Autodesk Inventor part; units mm, degrees
ref_plane "YZ Plane" through (0, 0, 0) normal (1, 0, 0) x (0, 1, 0)
ref_plane "XZ Plane" through (0, 0, 0) normal (0, 1, 0) x (-1, 0, 0)
ref_plane "XY Plane" through (0, 0, 0) normal (0, 0, 1) x (1, 0, 0)
sketch "Sketch1" plane through (0, 0, 0) normal (0, 0, 1) x (1, 0, 0)
  circle A0 centre (0, 0) radius 0.5
  circle A1 centre (-2.7681, 0.2813) radius 0.75
  circle A2 centre (-0.5, 7.6342) radius 1
  circle A3 centre (-0.5, 2.9376) radius 1.25
  circle A4 centre (-1.2054, -3.5313) radius 1.5
  circle A5 centre (-6.7502, -2.5313) radius 2.5
  circle A6 centre (-6.2681, 5.1832) radius 3.5
  line L0 (2.4912, -6.5091) -> (-11.3709, -6.5091)
  line L1 (-11.3709, -6.5091) -> (-11.3709, 10.0048)
  line L2 (-11.3709, 10.0048) -> (2.4912, 10.0048)
  line L3 (2.4912, 10.0048) -> (2.4912, -6.5091)
  dimension "d0" = 1
  dimension "d1" = 1.5
  dimension "d2" = 2
  dimension "d3" = 2.5
  dimension "d4" = 3
  dimension "d5" = 5
  dimension "d6" = 7
extrude "Extrusion1" add sketch "Sketch1" along normal blind 2
properties part number "hole_test"
The model under review builds one solid part; all positions refer to its coordinate system, in mm. Give positions to 0.01 mm unless a question says otherwise; leave off trailing zeros. Loops run counter-clockwise (first coordinate to the right, second up) from the corner with the lowest first, then second, coordinate; pieces in that order, holes last. Notation, with made-up numbers: (80, -31.5) -> (109, -31.5) arc R20 ccw to (109, 6.5) -> close; hole circle Ø9 at (30.25, -25.5). An arc over 180 degrees is marked (long way). Put each result on its own line as item: value. Start each with the question number.
1. Mouldability with a two-part tool opening along Y and no side actions: class faces 1 (the face through (0, 8.5, 1)), 2 (the face through (-5, 10.005, 1)), 3 (the face through (-11.371, 2, 1)) as released by +Y, released by -Y, zero draft, split by the parting line, or undercut.
2. Clearance check with a flat-ended pin moving along its axis: P1, Ø6.5, axis at x = -6.27, y = 5.18, coming from the +Z side. State where the tip first meets the part, or that it passes through.
3. We need section A-A on y = -2.25. State the section outline as (x, z) points, then the cut area to 3 significant figures.
4. We need section D-D on z = 0.65. State the section outline as (x, y) points, then the cut area to 3 significant figures.
5. We need section B-B on x = 0. State the section outline as (y, z) points.
6. We need section C-C on x = -3. State the section outline as (y, z) points, then the cut area to 3 significant figures.
7. Wall thickness on probe 1 along Y at (x, z) = (-5.25, 1.85); probe 2 along X at (y, z) = (5, 1.05); probe 3 along Y at (x, z) = (-7, 1.35): over which ranges is each line inside the solid? List them lowest first.
Determined:
1. face 1: undercut
1. face 2: released by +Y
1. face 3: zero draft
2. P1: through
3. outline: (-11.37, 0) -> (-9.23, 0) -> (-9.23, 2) -> (-11.37, 2) -> close; (-4.27, 0) -> (-1.99, 0) -> (-1.99, 2) -> (-4.27, 2) -> close; (-0.43, 0) -> (2.49, 0) -> (2.49, 2) -> (-0.43, 2) -> close
3. area: 14.7 mm^2
4. outline: (-11.37, -6.51) -> (2.49, -6.51) -> (2.49, 10) -> (-11.37, 10) -> close; hole circle Ø7 at (-6.27, 5.18); hole circle Ø5 at (-6.75, -2.53); hole circle Ø1.5 at (-2.77, 0.28); hole circle Ø3 at (-1.21, -3.53); hole circle Ø2.5 at (-0.5, 2.94); hole circle Ø2 at (-0.5, 7.63); hole circle Ø1 at (0, 0)
4. area: 153 mm^2
5. outline: (-6.51, 0) -> (-4.42, 0) -> (-4.42, 2) -> (-6.51, 2) -> close; (-2.64, 0) -> (-0.5, 0) -> (-0.5, 2) -> (-2.64, 2) -> close; (0.5, 0) -> (1.79, 0) -> (1.79, 2) -> (0.5, 2) -> close; (4.08, 0) -> (6.77, 0) -> (6.77, 2) -> (4.08, 2) -> close; (8.5, 0) -> (10, 0) -> (10, 2) -> (8.5, 2) -> close
6. outline: (-6.51, 0) -> (-0.43, 0) -> (-0.43, 2) -> (-6.51, 2) -> close; (0.99, 0) -> (3.93, 0) -> (3.93, 2) -> (0.99, 2) -> close; (6.44, 0) -> (10, 0) -> (10, 2) -> (6.44, 2) -> close
6. area: 25.2 mm^2
7. probe 1: -6.51 to -4.53, -0.53 to 1.83, 8.53 to 10
7. probe 2: -11.37 to -9.76, -2.77 to 2.49
7. probe 3: -6.51 to -5.02, -0.04 to 1.76, 8.61 to 10
